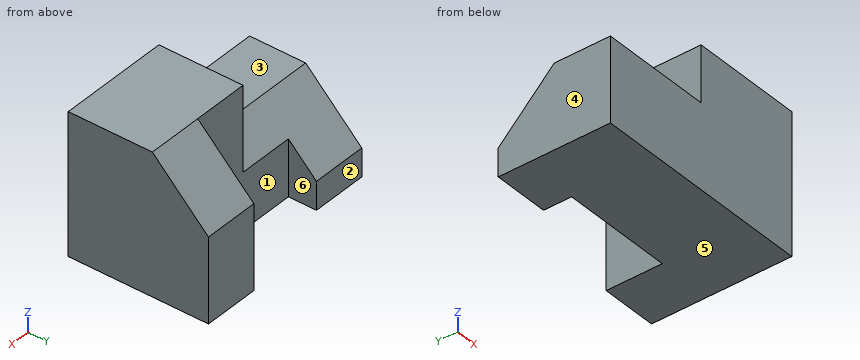
```python
from build123d import *

# Parameters (mm, degrees)
SKETCH1_W           = 80
SKETCH1_H           = 50
BOSS_EXTRUDE1_DEPTH = 30
SKETCH2_W           = 40
SKETCH2_H           = 20
CUT_EXTRUDE1_DEPTH  = 30
SKETCH3_W           = 20
SKETCH3_H           = 50
BOSS_EXTRUDE2_DEPTH = 20
CUT_EXTRUDE2_DEPTH  = 20
CUT_EXTRUDE4_DEPTH  = 40
BOSS_EXTRUDE3_DEPTH = 20


with BuildPart() as part:
    # Sketch1 → Boss-Extrude1 (new body)
    with BuildSketch(Plane(origin=(0, 0, 0), x_dir=(1, 0, 0), z_dir=(0, 1, 0))):
        with Locations((40, 25)):
            Rectangle(SKETCH1_W, SKETCH1_H)
    extrude(amount=BOSS_EXTRUDE1_DEPTH)

    # Sketch2 → Cut-Extrude1 (cut)
    with BuildSketch(Plane(origin=(0, 30, 0), x_dir=(1, 0, 0), z_dir=(0, 1, 0))):
        with Locations((20, 10)):
            Rectangle(SKETCH2_W, SKETCH2_H)
    extrude(amount=-CUT_EXTRUDE1_DEPTH, mode=Mode.SUBTRACT)

    # Sketch3 → Boss-Extrude2 (add)
    with BuildSketch(Plane(origin=(0, 30, 0), x_dir=(1, 0, 0), z_dir=(0, 1, 0))):
        with Locations((70, 25)):
            Rectangle(SKETCH3_W, SKETCH3_H)
    extrude(amount=BOSS_EXTRUDE2_DEPTH)

    # Sketch4 → Cut-Extrude2 (cut)
    with BuildSketch(Plane(origin=(80, 0, 0), x_dir=(0, 0, -1), z_dir=(1, 0, 0))):
        Polygon((20, 50), (0, 30), (0, 50), align=None)
    extrude(amount=-CUT_EXTRUDE2_DEPTH, mode=Mode.SUBTRACT)

    # Sketch5 → Cut-Extrude4 (cut)
    with BuildSketch(Plane.ZY):
        Polygon((-30, 30), (-20, 20), (-20, 30), align=None)
    extrude(amount=-CUT_EXTRUDE4_DEPTH, mode=Mode.SUBTRACT)

    # Sketch6 → Boss-Extrude3 (add)
    with BuildSketch(Plane.ZY):
        Polygon((-50, 30), (-50, 40), (-40, 40), (-30, 30), (-20, 20), (-20, 0), (-50, 0), align=None)
    extrude(amount=-BOSS_EXTRUDE3_DEPTH)


solid = part.part
```
Verification items for the finished model (mm, model axes). Face numbers are marked on the shaded views. A direction names the side the tool comes from. Coordinates: 2 decimals unless noted, no trailing zeros. Order: outer loops, then holes, each group sorted by start corner. A loop starts at its lowest first (then second) coordinate and runs counter-clockwise, first axis right, second up. Notation, with made-up numbers: (44, -39) - (94, -39) arc R32 cw to (94, -12) - close; hole circle Ø7 at (58, 7). An arc over 180 degrees is marked (long way). Return JSON: item names as keys, results as strings.
(1) Section check A-A, the plane y = 38. Record the cut outline in (x, z).
Filled sheet:
{"outline": "(0, -50) - (20, -50) - (20, -38) - (0, -38) - close; (60, -50) - (80, -50) - (80, -8) - (60, -8) - close"}
(2) Section check D-D, the plane y = 18. Record the cut outline in (x, z).
Filled sheet:
{"outline": "(0, -50) - (80, -50) - (80, 0) - (40, 0) - (40, -20) - (0, -20) - close"}
(3) Section check B-B, the plane z = -29. Record the cut outline in (x, y), and give its area (3 significant figures).
Filled sheet:
{"outline": "(0, 0) - (80, 0) - (80, 50) - (60, 50) - (60, 30) - (40, 30) - (40, 29) - (0, 29) - close", "area": "2,760 mm^2"}
(4) Section check C-C, the plane x = 9. Record the cut outline in (y, z).
Filled sheet:
{"outline": "(0, -50) - (40, -50) - (40, -40) - (20, -20) - (0, -20) - close"}
(5) Access from +Z, -Z, +X, -X, +Y, -Y to the whole of each face (thin tool, end or side, straight path). Record for the marked faces 1, 2 and 3.
Filled sheet:
{"face 1": "+Z, -Z, +Y", "face 2": "+Z, -Z, -X, +Y", "face 3": "+Z, -X, +Y, -Y"}
(6) Thickness scan on line 1 along Y through (x, z) = (11, -41.5); line 2 along Z through (x, y) = (39, 6); line 3 along Y through (x, z) = (50.5, -26.5). Record the ranges inside material, lowest first.
Filled sheet:
{"line 1": "y = 0 to 40", "line 2": "z = -50 to -20", "line 3": "y = 0 to 30"}
(7) Go/stop test with flat-tipped pins: pin 1 (1 mm diameter, centred on x = 13, y = 27, fed in from +Z); pin 2 (20 mm diameter, centred on x = 37.5, z = -27.5, fed in from +Y); pin 3 (8 mm diameter, centred on x = 13, z = -45.5, fed in from +Y). Record where each tip stops, or that it passes through.
Filled sheet:
{"pin 1": "stops at z = -26.5", "pin 2": "stops at y = 30", "pin 3": "stops at y = 40"}
(8) Mould release check, pull along X, two halves, no side actions. Record for the marked faces 4, 5 and 6: pulls with the +X half, pulls with the -X half, needs draft (parallel to the pull), parting line crosses it, or undercut.
Filled sheet:
{"face 4": "pulls with the -X half", "face 5": "needs draft", "face 6": "undercut"}
